```python
from build123d import *

# Parameters (mm, degrees)
BOSS_EXTRUDE1_DEPTH = 62
SKETCH2_R           = 6.829046467
BOSS_EXTRUDE2_DEPTH = 26
BOSS_EXTRUDE3_DEPTH = 19


with BuildPart() as part:
    # Sketch1 → Boss-Extrude1 (new body)
    with BuildSketch(Plane.XY):
        Polygon((0, 0), (0, 48.281138127), (26.053837569, 48.281138127), (55.644011692, 23.446527703), (55.644011692, 0), align=None)
    extrude(amount=BOSS_EXTRUDE1_DEPTH)

    # Sketch2 → Boss-Extrude2 (add)
    with BuildSketch(Plane(origin=(34.542354114, 41.156847455, 0), x_dir=(0.765974254, -0.642871249, 0), z_dir=(0.642871249, 0.765974254, 0))):
        with Locations((3.286422452, -32.740977781)):
            Circle(SKETCH2_R)
    extrude(amount=BOSS_EXTRUDE2_DEPTH)

    # Sketch3 → Boss-Extrude3 (add)
    with BuildSketch(Plane(origin=(51.257006582, 61.072178055, 0), x_dir=(0.765974254, -0.642871249, 0), z_dir=(0.642871249, 0.765974254, 0))):
        with BuildLine():
            Line((6.231595343, -34.685018308), (0.758276941, -33.629675248))
            ThreePointArc((0.758276941, -33.629675248), (-0.542233107, -31.707846996), (1.379595145, -30.407336949))
            Line((1.379595145, -30.407336949), (6.852913547, -31.462680009))
            ThreePointArc((6.852913547, -31.462680009), (8.153423595, -33.38450826), (6.231595343, -34.685018308))
        make_face()
    extrude(amount=BOSS_EXTRUDE3_DEPTH)


solid = part.part
```
The listing builds one solid part. Answer for the finished solid, in the listing's coordinates (mm). A direction names the side the tool comes from. Coordinates: 2 decimals unless noted, no trailing zeros. Order: outer loops, then holes, each group sorted by start corner. A loop starts at its lowest first (then second) coordinate and runs counter-clockwise, first axis right, second up. Notation, with made-up numbers: M 35.25,-33 L 68.25,-33 A16 ccw 68.25,-13 Z; hole C -2,-32.75 d8. An arc over 180 degrees is marked long. Answer as a JSON object with one key per item and string values. Group by question number.
1. Flat-ended cylindrical pins translate along their axes: P1, Ø7, axis at y = 15, z = 46, coming from the +X side; P2, Ø4, axis at x = 42.5, z = 9.5, coming from the +Y side; P3, Ø4, axis at x = 24.5, z = 23.5, coming from the +Y side. Find the tip coordinate at first contact, or state that the pin passes through.
2. Straight lines are drawn through the part: line 1 (Y direction, x = 13, z = 25); line 2 (X direction, y = 22.5, z = 37.5); line 3 (Z direction, x = 55.5, y = 51.5). For each, find the intervals that lie inside material, in ascending order.
3. Section C-C on x = 22.5 is taken. Write down the section's boundary in (y, z).
4. A tool of negligible diameter and unlimited length cuts with its end or side. For faces 1 (the flat face through (13, 48.281, 31)), 2 (the flat face through (55.644, 12, 31)), 3 (the flat face through (60.402, 65.625, 30.928)), 4 (the flat face through (59.985, 65.976, 34.165)), from which of +Z, -Z, +X, -X, +Y, -Y can it reach the whole face along a straight path? Write none if from no direction.
5. Section B-B on y = 17 is taken. Write down the section's boundary in (x, z).
6. Section D-D on z = 37 is taken. Write down the section's boundary in (x, y), then the cut area to 3 significant figures.
7. Section A-A on z = 58 is taken. Write down the section's boundary in (x, y).
Values follow:
{
 "1": {"P1": "x = 55.64", "P2": "y = 36.16", "P3": "y = 48.28"},
 "2": {"line 1": "0 to 48.28", "line 2": "0 to 55.64", "line 3": "29.71 to 35.78"},
 "3": {"outline": "M 0,0 L 48.28,0 L 48.28,62 L 0,62 Z"},
 "4": {"face 1": "+Z, -Z, -X, +Y", "face 2": "+Z, -Z, +X, -Y", "face 3": "-Z, +X", "face 4": "+Z, +Y"},
 "5": {"outline": "M 0,0 L 55.64,0 L 55.64,62 L 0,62 Z"},
 "6": {"outline": "M 0,0 L 55.64,0 L 55.64,23.45 L 41.15,35.61 L 57.86,55.53 L 49.69,62.39 L 32.97,42.48 L 26.05,48.28 L 0,48.28 Z", "area": "2,600 mm2"},
 "7": {"outline": "M 0,0 L 55.64,0 L 55.64,23.45 L 26.05,48.28 L 0,48.28 Z"}
}
